```python
from build123d import *

# Parameters (mm, degrees)
F0_R      = 6.5
F1_DEPTH  = 6.35
F2_SIZE   = 2.54
F4_DEPTH  = 304.8
F5_R      = 12.7
F6_R      = 25.4
F8_DEPTH  = 76.2
F9_R      = 25.4
F10_R     = 6.5
F11_DEPTH = 247.651


with BuildPart() as f1:
    # F0 (on Top) → F1 (new body)
    with BuildSketch(Plane.XY):
        with BuildLine():
            ThreePointArc((0, 25.4), (7.439488, 7.439488), (25.4, 0))
            Line((25.4, 0), (279.4, 0))
            ThreePointArc((279.4, 0), (297.360512, 7.439488), (304.8, 25.4))
            Line((304.8, 25.4), (304.8, 76.2))
            Line((304.8, 76.2), (0, 76.2))
            Line((0, 76.2), (0, 25.4))
        make_face()
        with Locations((27.94, 19.05)):
            Circle(F0_R, mode=Mode.SUBTRACT)
        with Locations((55.88, 19.05)):
            Circle(F0_R, mode=Mode.SUBTRACT)
        with Locations((83.82, 19.05)):
            Circle(F0_R, mode=Mode.SUBTRACT)
        with Locations((111.76, 19.05)):
            Circle(F0_R, mode=Mode.SUBTRACT)
        with Locations((139.7, 19.05)):
            Circle(F0_R, mode=Mode.SUBTRACT)
        with Locations((167.64, 19.05)):
            Circle(F0_R, mode=Mode.SUBTRACT)
        with Locations((195.58, 19.05)):
            Circle(F0_R, mode=Mode.SUBTRACT)
        with Locations((223.52, 19.05)):
            Circle(F0_R, mode=Mode.SUBTRACT)
        with Locations((251.46, 19.05)):
            Circle(F0_R, mode=Mode.SUBTRACT)
        with Locations((279.4, 19.05)):
            Circle(F0_R, mode=Mode.SUBTRACT)
        with Locations((27.94, 57.15)):
            Circle(F0_R, mode=Mode.SUBTRACT)
        with Locations((55.88, 57.15)):
            Circle(F0_R, mode=Mode.SUBTRACT)
        with Locations((83.82, 57.15)):
            Circle(F0_R, mode=Mode.SUBTRACT)
        with Locations((111.76, 57.15)):
            Circle(F0_R, mode=Mode.SUBTRACT)
        with Locations((139.7, 57.15)):
            Circle(F0_R, mode=Mode.SUBTRACT)
        with Locations((167.64, 57.15)):
            Circle(F0_R, mode=Mode.SUBTRACT)
        with Locations((195.58, 57.15)):
            Circle(F0_R, mode=Mode.SUBTRACT)
        with Locations((223.52, 57.15)):
            Circle(F0_R, mode=Mode.SUBTRACT)
        with Locations((251.46, 57.15)):
            Circle(F0_R, mode=Mode.SUBTRACT)
        with Locations((279.4, 57.15)):
            Circle(F0_R, mode=Mode.SUBTRACT)
    extrude(amount=F1_DEPTH)

    # F2
    f2_edges = [f1.edges().sort_by_distance(p)[0] for p in [
        (7.439488, 7.439488, 6.35),
        (152.4, 0, 6.35),
        (297.360512, 7.439488, 6.35),
        (304.8, 50.8, 6.35),
        (152.4, 76.2, 6.35),
        (0, 50.8, 6.35),
        (21.44, 19.05, 6.35),
        (49.38, 19.05, 6.35),
        (77.32, 19.05, 6.35),
        (105.26, 19.05, 6.35),
        (133.2, 19.05, 6.35),
        (161.14, 19.05, 6.35),
        (189.08, 19.05, 6.35),
        (217.02, 19.05, 6.35),
        (244.96, 19.05, 6.35),
        (272.9, 19.05, 6.35),
        (21.44, 57.15, 6.35),
        (49.38, 57.15, 6.35),
        (77.32, 57.15, 6.35),
        (105.26, 57.15, 6.35),
        (133.2, 57.15, 6.35),
        (161.14, 57.15, 6.35),
        (189.08, 57.15, 6.35),
        (217.02, 57.15, 6.35),
        (244.96, 57.15, 6.35),
        (272.9, 57.15, 6.35),
    ]]
    chamfer(f2_edges, length=F2_SIZE)

    # F3 (on Right) → F4 (join)
    with BuildSketch(Plane.YZ):
        Polygon((76.2, 254), (76.2, 0), (76.2, -50.8), (0, -50.8), (0, -57.15), (82.55, -57.15), (82.55, 254), align=None)
    extrude(amount=F4_DEPTH)

    # F5
    f5_edges = [f1.edges().sort_by_distance(p)[0] for p in [
        (152.4, 76.2, -50.8),
        (152.4, 82.55, -57.15),
    ]]
    fillet(f5_edges, radius=F5_R)

    # F6
    f6_edges = [f1.edges().sort_by_distance(p)[0] for p in [
        (304.8, 79.375, 254),
        (0, 79.375, 254),
    ]]
    fillet(f6_edges, radius=F6_R)

    # F7 (on face) → F8 (join)
    with BuildSketch(Plane.XZ.offset(-76.2)):
        Polygon((304.8, 107.95), (0, 209.55), (-2.008047, 203.52586), (302.791953, 101.92586), align=None)
    extrude(amount=F8_DEPTH)

    # F9
    f9_edges = [f1.edges().sort_by_distance(p)[0] for p in [
        (304.8, 0, -53.975),
        (0, 0, -53.975),
        (-1.004023, 0, 206.53793),
        (303.795977, 0, 104.93793),
    ]]
    fillet(f9_edges, radius=F9_R)

    # F10 (on face) → F11 (cut, through all)
    with BuildSketch(Plane.XY.offset(6.35)):
        with Locations((27.94, 57.15)):
            Circle(F10_R)
        with Locations((27.94, 19.05)):
            Circle(F10_R)
        with Locations((55.88, 57.15)):
            Circle(F10_R)
        with Locations((55.88, 19.05)):
            Circle(F10_R)
        with Locations((83.82, 57.15)):
            Circle(F10_R)
        with Locations((111.76, 57.15)):
            Circle(F10_R)
        with Locations((83.82, 19.05)):
            Circle(F10_R)
        with Locations((111.76, 19.05)):
            Circle(F10_R)
        with Locations((139.7, 19.05)):
            Circle(F10_R)
        with Locations((139.7, 57.15)):
            Circle(F10_R)
        with Locations((167.64, 57.15)):
            Circle(F10_R)
        with Locations((167.64, 19.05)):
            Circle(F10_R)
        with Locations((195.58, 19.05)):
            Circle(F10_R)
        with Locations((195.58, 57.15)):
            Circle(F10_R)
        with Locations((223.52, 57.15)):
            Circle(F10_R)
        with Locations((223.52, 19.05)):
            Circle(F10_R)
        with Locations((251.46, 57.15)):
            Circle(F10_R)
        with Locations((251.46, 19.05)):
            Circle(F10_R)
        with Locations((279.4, 57.15)):
            Circle(F10_R)
        with Locations((279.4, 19.05)):
            Circle(F10_R)
    extrude(amount=F11_DEPTH, mode=Mode.SUBTRACT)


solid = f1.part
```
Here's how the part is built. I have some questions about the finished solid (model axes, mm). A direction names the side the tool comes from. Coordinates: 2 decimals unless noted, no trailing zeros. Order: outer loops, then holes, each group sorted by start corner. A loop starts at its lowest first (then second) coordinate and runs counter-clockwise, first axis right, second up.
1) Which directions (+Z, -Z, +X, -X, +Y, -Y) give clear straight access to the entire face, cutting with the end or side of a thin tool? Please do faces 1 (the face through (226.519, 13.283, 131.664)), 2 (the face through (150, 39, 0)), 3 (the face through (7.24, 7.64, -54.02)), 4 (the face through (246.176, 53.098, 3.969)).
2) Imagine slicing it at B-B on x = 195.58. State how many separate pieces and enclosed holes the cut face has, and give its area (3 significant figures).
3) I need wall thicknesses on line 1 (Y direction, x = 279, z = 114); line 2 (Z direction, x = 78.5, y = 41); line 3 (Z direction, x = 32.5, y = 52). Which ranges of each line are inside material? Lowest first, please.
4) Will these pins go through, and if not, where does the flat tip stop? pin 1 (6 mm diameter, centred on y = 54, z = 136.5, fed in from +X); pin 2 (21 mm diameter, centred on x = 167.64, y = 57.15, fed in from +Z); pin 3 (11.5 mm diameter, centred on x = 279.4, y = 19.05, fed in from +Z).
5) Imagine slicing it at A-A on z = -5. List the corners of the cut face in (x, y) for me.
6) We'd pull the mould along X, two halves only. Please class faces 5 (the face through (148.258, 38.633, 153.437)), 6 (the face through (285.6, 59.1, 1.9)), 7 (the face through (297.56, 7.64, -54.02)): +X half, -X half, draft (parallel to the pull), parting line (faces both ways), or undercut.
Response values:
1. face 1: +Z
1. face 2: +X, -X, -Y
1. face 3: -Z, -X, -Y
1. face 4: none
2. separate pieces: 5
2. enclosed holes: 0
2. area: 3,100 mm2
3. line 1: y = 0 to 12.56, 25.54 to 50.66, 63.64 to 82.55
3. line 2: z = -57.15 to -50.8, 0 to 6.35, 176.69 to 183.38
3. line 3: z = -57.15 to -50.8, 0 to 4.19, 192.02 to 198.72
4. pin 1: stops at x = 221.2
4. pin 2: stops at z = 157.17
4. pin 3: stops at z = -50.8
5. outline: (0, 76.2) - (304.8, 76.2) - (304.8, 82.55) - (0, 82.55) - close
6. face 5: -X half
6. face 6: undercut
6. face 7: +X half
